from build123d import *

# Parameters (mm, degrees)
F1_DEPTH = 55.626
F2_R     = 5.08
F3_DEPTH = 2.794
F4_R     = 3.175
F5_R     = 10.770919
F6_DEPTH = 3.81
F7_R     = 12.796254
F8_DEPTH = 8.89


with BuildPart() as f1:
    # F0 (on Top) → F1 (new body)
    with BuildSketch(Plane.XY):
        with BuildLine():
            ThreePointArc((-17.4625, -7.9375), (-15.602628, -12.427628), (-11.1125, -14.2875))
            Line((-11.1125, -14.2875), (11.1125, -14.2875))
            ThreePointArc((11.1125, -14.2875), (15.602628, -12.427628), (17.4625, -7.9375))
            Line((17.4625, -7.9375), (17.4625, 7.9375))
            ThreePointArc((17.4625, 7.9375), (15.602628, 12.427628), (11.1125, 14.2875))
            Line((11.1125, 14.2875), (-11.1125, 14.2875))
            ThreePointArc((-11.1125, 14.2875), (-15.602628, 12.427628), (-17.4625, 7.9375))
            Line((-17.4625, 7.9375), (-17.4625, -7.9375))
        make_face()
    extrude(amount=F1_DEPTH)

    # F2
    f2_edges = [f1.edges().sort_by_distance(p)[0] for p in [
        (15.602628, -12.427628, 55.626),
    ]]
    fillet(f2_edges, radius=F2_R)

    # F0 (on Top) → F3 (join)
    with BuildSketch(Plane.XY):
        with BuildLine():
            ThreePointArc((-17.4625, -7.9375), (-15.602628, -12.427628), (-11.1125, -14.2875))
            Line((-11.1125, -14.2875), (11.1125, -14.2875))
            ThreePointArc((11.1125, -14.2875), (15.602628, -12.427628), (17.4625, -7.9375))
            Line((17.4625, -7.9375), (17.4625, 7.9375))
            ThreePointArc((17.4625, 7.9375), (15.602628, 12.427628), (11.1125, 14.2875))
            Line((11.1125, 14.2875), (-11.1125, 14.2875))
            ThreePointArc((-11.1125, 14.2875), (-15.602628, 12.427628), (-17.4625, 7.9375))
            Line((-17.4625, 7.9375), (-17.4625, -7.9375))
        make_face()
    extrude(amount=-F3_DEPTH)

    # F4
    f4_edges = [f1.edges().sort_by_distance(p)[0] for p in [
        (-15.602628, -12.427628, -2.794),
    ]]
    fillet(f4_edges, radius=F4_R)

    # F5 (on face) → F6 (join)
    with BuildSketch(Plane.XY.offset(55.626)):
        Circle(F5_R)
    extrude(amount=F6_DEPTH)

    # F7 (on face) → F8 (join)
    with BuildSketch(Plane.XY.offset(59.436)):
        Circle(F7_R)
    extrude(amount=F8_DEPTH)


solid = f1.part
For this review, take the finished solid that the model builds, in its own axes (mm). A direction names the side the tool comes from. Round coordinates to 2 decimals unless told otherwise and drop trailing zeros. Write each loop counter-clockwise with the first axis right and the second up, starting at its lowest first coordinate (ties: lowest second). Pieces come first, ordered by that corner, then holes. Notation, with made-up numbers: (55, 50) - (74, 50) arc R31 ccw to (74, 75) - close; hole circle Ø6 at (83.5, -32). An arc over 180 degrees is marked (long way). Use a Markdown table: item, result.
Q1. Machinability: for faces 1 (the cylindrical face through (6.88, 10.79, 63.82)), 2 (the cylindrical face through (10.27, 3.24, 57.5)), 3 (the flat face through (17.462, 0, 26)), which of the approach directions +Z, -Z, +X, -X, +Y, -Y give a long, thin tool a straight path to every point of the face, cutting with its end or side? Answer none if there is none.
Derived:
| item | result |
|---|---|
| face 1 | +Z |
| face 2 | none |
| face 3 | +Z, -Z, +X, +Y, -Y |
Q2. Wall thickness on line 1 along Z through (x, y) = (11.5, 5.5); line 2 along Y through (x, z) = (11.5, 54.5); line 3 along Z through (x, y) = (-1, 11): over which ranges is each line inside the solid? List them lowest first.
Derived:
| item | result |
|---|---|
| line 1 | z = -2.79 to 55.63, 59.44 to 68.33 |
| line 2 | y = -12.38 to 12.38 |
| line 3 | z = -2.79 to 55.3, 59.44 to 68.33 |
Q3. We need section D-D (z = 57.5). Give the boundary of the cut face in (x, y).
Derived:
| item | result |
|---|---|
| outline | circle Ø21.54 at (0, 0) |
Q4. The part is to be moulded in two halves that separate along Z. For faces 4 (the cylindrical face through (-15.55, 12.48, 25.81)), 5 (the flat face through (0, 0, -2.794)), 6 (the cylindrical face through (0.16, -12.84, 54.1)), 7 (the flat face through (-5.7, -9.4, 59.436)), say which applies: pulls with the +Z half, pulls with the -Z half, needs draft (parallel to the pull), parting line crosses it, or undercut.
Derived:
| item | result |
|---|---|
| face 4 | needs draft |
| face 5 | pulls with the -Z half |
| face 6 | undercut |
| face 7 | undercut |
Q5. We need section C-C (z = 7.5). Give the boundary of the cut face in (x, y), plus the area to 3 significant figures.
Derived:
| item | result |
|---|---|
| outline | (-17.46, -7.94) arc R6.35 ccw to (-11.11, -14.29) - (11.11, -14.29) arc R6.35 ccw to (17.46, -7.94) - (17.46, 7.94) arc R6.35 ccw to (11.11, 14.29) - (-11.11, 14.29) arc R6.35 ccw to (-17.46, 7.94) - close |
| area | 963 mm2 |
